```python
from build123d import *

# Parameters (mm, degrees)
F1_DEPTH = 3.175


# Not quite as in the source:
# - a length typed as a fraction of an inch, garbled in the dataset ("3 / 203.2 mm" for 3/8 in), is restored


with BuildPart() as f1:
    # F0 (on Right) → F1 (new body)
    with BuildSketch(Plane.YZ):
        Polygon((16.0724163434, -25.675), (16.0724163434, -22.5), (22.4224163434, -22.5), (22.4224163434, 16.15), (16.0724163434, 16.15), (16.0724163434, 19.325), (6.0724163434, 19.325), (6.0724163434, 16.15), (-6.2275836566, 16.15), (-6.2275836566, 19.325), (-16.2275836566, 19.325), (-16.2275836566, 16.15), (-19.4025836566, 16.15), (-19.325, -22.5), (-16.0724163434, -22.5), (-16.0724163434, -25.675), (-6.0724163434, -25.675), (-6.0724163434, -24.0875), (-6.0724163434, -22.5), (6.0724163434, -22.5), (6.0724163434, -24.0875), (6.0724163434, -25.675), align=None)
        Polygon((-8.5875, 2.325), (-8.5875, -3.175), (-8.5875, -8.675), (-11.0875, -8.675), (-11.0875, 2.325), align=None, mode=Mode.SUBTRACT)
        Polygon((1.5875, -3.175), (1.5875, -7.175), (-1.5875, -7.175), (-1.5875, -3.175), (-1.5875, 0.825), (1.5875, 0.825), align=None, mode=Mode.SUBTRACT)
        Polygon((8.5875, -8.675), (8.5875, -3.175), (8.5875, 2.325), (11.0875, 2.325), (11.0875, -8.675), align=None, mode=Mode.SUBTRACT)
        Polygon((-22.5775836566, -22.5), (-19.325, -22.5), (-19.4025836566, 16.15), (-22.5775836566, 16.15), align=None)
    extrude(amount=F1_DEPTH)


solid = f1.part
```
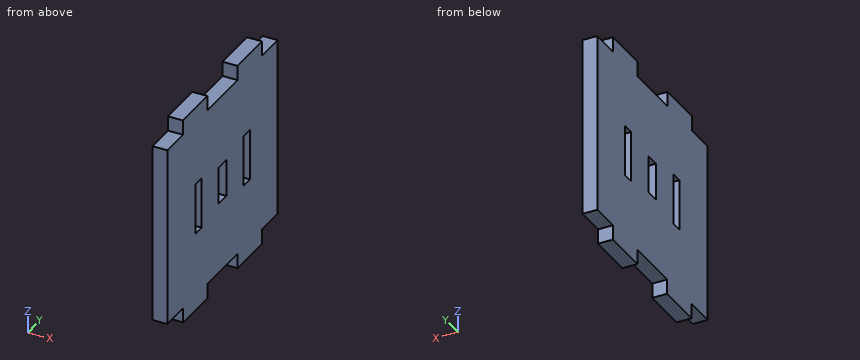
Could you check a few things on this model? Use its own coordinates, in mm. Coordinates: 2 decimals unless noted, no trailing zeros. Write each loop counter-clockwise with the first axis right and the second up, starting at its lowest first coordinate (ties: lowest second). Pieces come first, ordered by that corner, then holes. Notation, with made-up numbers: (59, -31.75) -> (98, -31.75) arc R16 ccw to (98, -14.75) -> close; hole circle Ø8 at (80.5, 25.5). An arc over 180 degrees is marked (long way). Write item = value, one per line. Start each with the question number.
(1) Will these pins go through, and if not, where does the flat tip stop? pin 1 (1.6 mm diameter, centred on x = 2, z = -24, fed in from -Y); pin 2 (1.6 mm diameter, centred on x = 2, z = 17.5, fed in from +Y).
(2) I need wall thicknesses on line 1 (Y direction, x = 0.2, z = -0.5); line 2 (Z direction, x = 3.05, y = -10.5) (3 decimals); line 3 (Y direction, x = 2.55, z = -24). Which ranges of each line are inside material? Lowest first, please. Write a range as [from, to].
(3) I want a section at B-B (y = 1). Please give me the cut outline in (x, z) (3 decimals).
(4) I want a section at A-A (x = 1.4). Give the number of separate pieces and of enclosed holes in the cut face, plus the area to 3 significant figures.
Result set:
q1.pin_1 = -16.07
q1.pin_2 = 16.07
q2.line_1 = [-22.58, -11.09], [-8.59, -1.59], [1.59, 8.59], [11.09, 22.42]
q2.line_2 = [-25.675, -8.675], [2.325, 19.325]
q2.line_3 = [-16.07, -6.07], [6.07, 16.07]
q3.outline = (0, -22.5) -> (3.175, -22.5) -> (3.175, -7.175) -> (0, -7.175) -> close; (0, 0.825) -> (3.175, 0.825) -> (3.175, 16.15) -> (0, 16.15) -> close
q4.separate_pieces = 1
q4.enclosed_holes = 3
q4.area = 1,790 mm2
